Autodesk Fusion 360 part; units mm, degrees
sketch "Sketch1" plane through (0, 0, 0) normal (0, 1, 0) x (1, 0, 0)
  line L0 (-97, 45) -> (97, 45)
  line L1 (100, 42) -> (100, -42)
  line L2 (97, -45) -> (-97, -45)
  line L3 (-100, -42) -> (-100, 42)
  line L4 (-100, 45) -> (100, -45) construction
  line L5 (100, 45) -> (-100, -45) construction
  arc A0 (-100, -42) -> (-97, -45) centre (-97, -42) ccw
  arc A1 (97, -45) -> (100, -42) centre (97, -42) ccw
  arc A2 (100, 42) -> (97, 45) centre (97, 42) ccw
  arc A3 (-97, 45) -> (-100, 42) centre (-97, 42) ccw
  line L6 (-94.4444, 10) -> (-75.6944, 10)
  line L7 (-75.6944, 10) -> (-75.6944, 35)
  line L8 (-75.6944, 35) -> (-94.4444, 35)
  line L9 (-94.4444, 35) -> (-94.4444, 10)
  line L10 (-70.1389, 10) -> (-51.3889, 10)
  line L11 (-70.1389, 35) -> (-70.1389, 10)
  line L12 (-51.3889, 10) -> (-51.3889, 35)
  line L13 (-51.3889, 35) -> (-70.1389, 35)
  line L14 (-45.8333, 10) -> (-27.0833, 10)
  line L15 (-45.8333, 35) -> (-45.8333, 10)
  line L16 (-27.0833, 10) -> (-27.0833, 35)
  line L17 (-27.0833, 35) -> (-45.8333, 35)
  line L18 (-21.5278, 10) -> (-2.7778, 10)
  line L19 (-21.5278, 35) -> (-21.5278, 10)
  line L20 (-2.7778, 10) -> (-2.7778, 35)
  line L21 (-2.7778, 35) -> (-21.5278, 35)
  line L22 (2.7778, 10) -> (21.5278, 10)
  line L23 (2.7778, 35) -> (2.7778, 10)
  line L24 (21.5278, 10) -> (21.5278, 35)
  line L25 (21.5278, 35) -> (2.7778, 35)
  line L26 (27.0833, 10) -> (45.8333, 10)
  line L27 (27.0833, 35) -> (27.0833, 10)
  line L28 (45.8333, 10) -> (45.8333, 35)
  line L29 (45.8333, 35) -> (27.0833, 35)
  line L30 (51.3889, 10) -> (70.1389, 10)
  line L31 (51.3889, 35) -> (51.3889, 10)
  line L32 (70.1389, 10) -> (70.1389, 35)
  line L33 (70.1389, 35) -> (51.3889, 35)
  line L34 (75.6944, 10) -> (94.4444, 10)
  line L35 (75.6944, 35) -> (75.6944, 10)
  line L36 (94.4444, 10) -> (94.4444, 35)
  line L37 (94.4444, 35) -> (75.6944, 35)
  line L38 (-81.58, -45) -> (-78.58, -45)
  line L39 (-78.58, -45) -> (-78.58, -4.5)
  line L40 (-78.58, -4.5) -> (-81.58, -4.5)
  line L41 (-81.58, -4.5) -> (-81.58, -45)
  line L42 (-60.16, -45) -> (-57.11, -45)
  line L43 (-57.11, -45) -> (-57.11, -4.5)
  line L44 (-57.11, -4.5) -> (-60.16, -4.5)
  line L45 (-60.16, -4.5) -> (-60.16, -45)
  line L46 (-38.69, -45) -> (-35.59, -45)
  line L47 (-35.59, -45) -> (-35.59, -4.5)
  line L48 (-35.59, -4.5) -> (-38.69, -4.5)
  line L49 (-38.69, -4.5) -> (-38.69, -45)
  line L50 (-17.17, -45) -> (-14.02, -45)
  line L51 (-14.02, -45) -> (-14.02, -4.5)
  line L52 (-14.02, -4.5) -> (-17.17, -4.5)
  line L53 (-17.17, -4.5) -> (-17.17, -45)
  line L54 (4.4, -45) -> (1.2, -45)
  line L55 (1.2, -45) -> (1.2, -4.5)
  line L56 (1.2, -4.5) -> (4.4, -4.5)
  line L57 (4.4, -4.5) -> (4.4, -45)
  line L58 (19.62, -45) -> (22.87, -45)
  line L59 (22.87, -45) -> (22.87, -4.5)
  line L60 (22.87, -4.5) -> (19.62, -4.5)
  line L61 (19.62, -4.5) -> (19.62, -45)
  line L62 (56.41, -45) -> (59.76, -45)
  line L63 (59.76, -45) -> (59.76, -4.5)
  line L64 (59.76, -4.5) -> (56.41, -4.5)
  line L65 (56.41, -4.5) -> (56.41, -45)
  line L66 (78.18, -45) -> (81.58, -45)
  line L67 (81.58, -45) -> (81.58, -4.5)
  line L68 (81.58, -4.5) -> (78.18, -4.5)
  line L69 (78.18, -4.5) -> (78.18, -45)
  line L70 (37.99, -45) -> (41.29, -45)
  line L71 (41.29, -45) -> (41.29, -4.5)
  line L72 (41.29, -4.5) -> (37.99, -4.5)
  line L73 (37.99, -4.5) -> (37.99, -45)
  line L74 (-100, -24.75) -> (-81.58, -24.75) construction
  line L75 (-57.11, -24.75) -> (-38.69, -24.75) construction
  line L76 (-35.59, -24.75) -> (-17.17, -24.75) construction
  line L77 (-14.02, -24.75) -> (4.4, -24.75) construction
  line L78 (1.2, -24.75) -> (19.62, -24.75) construction
  line L79 (22.87, -24.75) -> (41.29, -24.75) construction
  line L80 (37.99, -24.75) -> (56.41, -24.75) construction
  line L81 (59.76, -24.75) -> (78.18, -24.75) construction
  line L82 (81.58, -24.75) -> (100, -24.75) construction
  line L83 (-78.58, -24.75) -> (-60.16, -24.75) construction
  dimension "d8" = 3
  dimension "d9" = 90
  dimension "d10" = 200
  dimension "d16" = 5.5556
  dimension "d17" = 10
  dimension "d18" = 10
  dimension "d19" = 18.75
  dimension "d22" = 24.3056
  dimension "d23" = 0
  dimension "d24" = 3
  dimension "d25" = 40.5
  dimension "d26" = 3.05
  dimension "d27" = 3.1
  dimension "d28" = 3.15
  dimension "d29" = 3.2
  dimension "d30" = 3.25
  dimension "d31" = 3.3
  dimension "d32" = 3.35
  dimension "d33" = 3.4
extrude "Extrude1" add sketch "Sketch1" along normal blind 3 contours L0 L1 L2 L3 A0 A1 A2 A3 L39 L40 L41 L43 L44 L45 L47 L48 L49 L51 L52 L53 L55 L56 L57 L59 L60 L61 L63 L64 L65 L67 L68 L69 L71 L72 L73
fillet "Fillet1" radius 3 18 edges at (-81.58, 1.5, 45) (-78.58, 1.5, 45) (-60.16, 1.5, 45) (-57.11, 1.5, 45) (-35.59, 1.5, 45) (-38.69, 1.5, 45) (-14.02, 1.5, 45) (-17.17, 1.5, 45) (1.2, 1.5, 45) (4.4, 1.5, 45) (19.62, 1.5, 45) (22.87, 1.5, 45) (37.99, 1.5, 45) (41.29, 1.5, 45) (56.41, 1.5, 45) (59.76, 1.5, 45) (78.18, 1.5, 45) (81.58, 1.5, 45)
sketch "Sketch2" plane through (0, 0, 0) normal (0, -1, 0) x (1, 0, 0)
  line L0 (94.4444, -35) -> (75.6944, -35)
  line L1 (75.6944, -35) -> (75.6944, -10)
  line L2 (75.6944, -10) -> (94.4444, -10)
  line L3 (94.4444, -10) -> (94.4444, -35)
  line L4 (-94.4444, -35) -> (-94.4444, -10)
  line L5 (-94.4444, -10) -> (-75.6944, -10)
  line L6 (-75.6944, -10) -> (-75.6944, -35)
  line L7 (-75.6944, -35) -> (-94.4444, -35)
  line L8 (70.1389, -35) -> (51.3889, -35)
  line L9 (51.3889, -35) -> (51.3889, -10)
  line L10 (51.3889, -10) -> (70.1389, -10)
  line L11 (70.1389, -10) -> (70.1389, -35)
  line L12 (-2.7778, -35) -> (-21.5278, -35)
  line L13 (-21.5278, -35) -> (-21.5278, -10)
  line L14 (-21.5278, -10) -> (-2.7778, -10)
  line L15 (-2.7778, -10) -> (-2.7778, -35)
  line L16 (21.5278, -35) -> (2.7778, -35)
  line L17 (2.7778, -35) -> (2.7778, -10)
  line L18 (2.7778, -10) -> (21.5278, -10)
  line L19 (21.5278, -10) -> (21.5278, -35)
  line L20 (-51.3889, -35) -> (-70.1389, -35)
  line L21 (-70.1389, -35) -> (-70.1389, -10)
  line L22 (-70.1389, -10) -> (-51.3889, -10)
  line L23 (-51.3889, -10) -> (-51.3889, -35)
  line L24 (-27.0833, -35) -> (-45.8333, -35)
  line L25 (-45.8333, -35) -> (-45.8333, -10)
  line L26 (-45.8333, -10) -> (-27.0833, -10)
  line L27 (-27.0833, -10) -> (-27.0833, -35)
  line L28 (45.8333, -35) -> (27.0833, -35)
  line L29 (27.0833, -35) -> (27.0833, -10)
  line L30 (27.0833, -10) -> (45.8333, -10)
  line L31 (45.8333, -10) -> (45.8333, -35)
  arc A0 (84.58, 45) -> (81.58, 42) centre (84.58, 42) ccw
  line L32 (81.58, 42) -> (81.58, 4.5)
  line L33 (81.58, 4.5) -> (78.18, 4.5)
  line L34 (78.18, 4.5) -> (78.18, 42)
  arc A1 (78.18, 42) -> (75.18, 45) centre (75.18, 42) ccw
  line L35 (75.18, 45) -> (62.76, 45)
  arc A2 (62.76, 45) -> (59.76, 42) centre (62.76, 42) ccw
  line L36 (59.76, 42) -> (59.76, 4.5)
  line L37 (59.76, 4.5) -> (56.41, 4.5)
  line L38 (56.41, 4.5) -> (56.41, 42)
  arc A3 (56.41, 42) -> (53.41, 45) centre (53.41, 42) ccw
  line L39 (53.41, 45) -> (44.29, 45)
  arc A4 (44.29, 45) -> (41.29, 42) centre (44.29, 42) ccw
  line L40 (41.29, 42) -> (41.29, 4.5)
  line L41 (41.29, 4.5) -> (37.99, 4.5)
  line L42 (37.99, 4.5) -> (37.99, 42)
  arc A5 (37.99, 42) -> (34.99, 45) centre (34.99, 42) ccw
  line L43 (34.99, 45) -> (25.87, 45)
  arc A6 (25.87, 45) -> (22.87, 42) centre (25.87, 42) ccw
  line L44 (22.87, 42) -> (22.87, 4.5)
  line L45 (22.87, 4.5) -> (19.62, 4.5)
  line L46 (19.62, 4.5) -> (19.62, 42)
  arc A7 (19.62, 42) -> (16.62, 45) centre (16.62, 42) ccw
  line L47 (16.62, 45) -> (7.4, 45)
  arc A8 (7.4, 45) -> (4.4, 42) centre (7.4, 42) ccw
  line L48 (4.4, 42) -> (4.4, 4.5)
  line L49 (4.4, 4.5) -> (1.2, 4.5)
  line L50 (1.2, 4.5) -> (1.2, 42)
  arc A9 (1.2, 42) -> (-1.8, 45) centre (-1.8, 42) ccw
  line L51 (-1.8, 45) -> (-11.02, 45)
  arc A10 (-11.02, 45) -> (-14.02, 42) centre (-11.02, 42) ccw
  line L52 (-14.02, 42) -> (-14.02, 4.5)
  line L53 (-14.02, 4.5) -> (-17.17, 4.5)
  line L54 (-17.17, 4.5) -> (-17.17, 42)
  arc A11 (-17.17, 42) -> (-20.17, 45) centre (-20.17, 42) ccw
  line L55 (-20.17, 45) -> (-32.59, 45)
  arc A12 (-32.59, 45) -> (-35.59, 42) centre (-32.59, 42) ccw
  line L56 (-35.59, 42) -> (-35.59, 4.5)
  line L57 (-35.59, 4.5) -> (-38.69, 4.5)
  line L58 (-38.69, 4.5) -> (-38.69, 42)
  arc A13 (-38.69, 42) -> (-41.69, 45) centre (-41.69, 42) ccw
  line L59 (-41.69, 45) -> (-54.11, 45)
  arc A14 (-54.11, 45) -> (-57.11, 42) centre (-54.11, 42) ccw
  line L60 (-57.11, 42) -> (-57.11, 4.5)
  line L61 (-57.11, 4.5) -> (-60.16, 4.5)
  line L62 (-60.16, 4.5) -> (-60.16, 42)
  arc A15 (-60.16, 42) -> (-63.16, 45) centre (-63.16, 42) ccw
  line L63 (-63.16, 45) -> (-75.58, 45)
  arc A16 (-75.58, 45) -> (-78.58, 42) centre (-75.58, 42) ccw
  line L64 (-78.58, 42) -> (-78.58, 4.5)
  line L65 (-78.58, 4.5) -> (-81.58, 4.5)
  line L66 (-81.58, 4.5) -> (-81.58, 42)
  arc A17 (-81.58, 42) -> (-84.58, 45) centre (-84.58, 42) ccw
  line L67 (-84.58, 45) -> (-97, 45)
  arc A18 (-97, 45) -> (-100, 42) centre (-97, 42) ccw
  line L68 (-100, 42) -> (-100, -42)
  arc A19 (-100, -42) -> (-97, -45) centre (-97, -42) ccw
  line L69 (-97, -45) -> (97, -45)
  arc A20 (97, -45) -> (100, -42) centre (97, -42) ccw
  line L70 (100, -42) -> (100, 42)
  arc A21 (100, 42) -> (97, 45) centre (97, 42) ccw
  line L71 (97, 45) -> (84.58, 45)
equation "Wbox = 200 mm"
equation "Hbox = 90 mm"
equation "Thickness = 3 mm"
equation "Kerfincrement = 0.05 mm"
equation "Diameter = 5 mm"
equation "Fillet = 3 mm"
equation "Kerfsteps = 6 mm"
equation "d8 = Fillet"
equation "d9 = Hbox"
equation "d10 = Wbox"
equation "PSwidth = ( Wbox * 0.75 ) / PScount"
equation "PSgap = ( Wbox - ( PSwidth * PScount ) ) / ( PScount + 1 )"
equation "d16 = PSgap"
equation "d17 = Wbox * 0.05"
equation "d18 = Wbox * 0.05"
equation "d19 = PSwidth"
equation "d22 = PSwidth + PSgap"
equation "d24 = Thickness"
equation "d25 = 0.45 * Hbox"
equation "d26 = Thickness + ( 1 * Kerfincrement )"
equation "d27 = Thickness + ( 2 * Kerfincrement )"
equation "d28 = Thickness + ( 3 * Kerfincrement )"
equation "d29 = Thickness + ( 4 * Kerfincrement )"
equation "d30 = Thickness + ( 5 * Kerfincrement )"
equation "d31 = Thickness + ( 6 * Kerfincrement )"
equation "d32 = Thickness + ( 7 * Kerfincrement )"
equation "d33 = Thickness + ( 8 * Kerfincrement )"
equation "d34 = Thickness"
equation "d37 = Fillet"
Input: part model. Units: mm. Frame: model coordinates. Give positions to 0.01 mm unless a question says otherwise; leave off trailing zeros. Loops run counter-clockwise (first coordinate to the right, second up) from the corner with the lowest first, then second, coordinate; pieces in that order, holes last. Notation, with made-up numbers: (83, 41.5) -> (125, 41.5) arc R5 ccw to (125, 49.5) -> close; hole circle Ø11 at (76, 39). An arc over 180 degrees is marked (long way). Answer as a JSON object with one key per item and string values. Group by question number.
Item 1: Cut plane B-B, the plane y = 0.55. State how many separate pieces and enclosed holes the cut face has, and give its area (3 significant figures).
Item 2: Pin query (flat end, axial travel): P1, Ø1.5, axis at x = -58, y = 1, coming from the +Z side. Return the tip coordinate at first contact, or that it passes through.
Item 3: Pull-direction query (Y, two-part tool) for faces 1 (the flat face through (-1, 0, -1)), 2 (the flat face through (-1, 3, -1)); classes: released by +Y, released by -Y, zero draft, split by the parting line, or undercut.
Item 4: Line query: probe 1 along Z at (x, y) = (-79, 1.8); probe 2 along Z at (x, y) = (15.5, 0.35). Output: solid intervals per line, ascending.
Item 5: Cut plane A-A, the plane x = -65. Return the cut outline in (y, z).
Checks:
{
 "1": {"separate pieces": "1", "enclosed holes": "8", "area": "13,000 mm²"},
 "2": {"P1": "stops at z = 4.5"},
 "3": {"face 1": "released by -Y", "face 2": "released by +Y"},
 "4": {"probe 1": "z = -45 to -35, -10 to 4.5", "probe 2": "z = -45 to -35, -10 to 45"},
 "5": {"outline": "(0, -45) -> (3, -45) -> (3, -35) -> (0, -35) -> close; (0, -10) -> (3, -10) -> (3, 45) -> (0, 45) -> close"}
}
